Check sheet for the modelled part. Datum: model origin and axes. Units: mm. A direction names the side the tool comes from. Give positions to 0.01 mm unless a question says otherwise; leave off trailing zeros. Loops run counter-clockwise (first coordinate to the right, second up) from the corner with the lowest first, then second, coordinate; pieces in that order, holes last. Notation, with made-up numbers: (-27, 42) -> (-3, 42) arc R9 ccw to (-3, 51) -> close; hole circle Ø4 at (28, -16.75). An arc over 180 degrees is marked (long way). Write each question's results on one line, items separated by ' | '. Start each with the question number.
Item 1: Access from +Z, -Z, +X, -X, +Y, -Y to the whole of each face (thin tool, end or side, straight path). Record for faces 5 (the face through (-0.96, -8.87, -4.34)), 6 (the face through (-8.807, -14.829, 3.935)).
Item 2: Mould release check, pull along X, two halves, no side actions. Record for faces 1 (the face through (-5, -17.018, 5)), 2 (the face through (-1.38, -21.15, -6.2)), 3 (the face through (3, -12.7, -6)), 4 (the face through (2.264, -14.829, 10.412)): pulls with the +X half, pulls with the -X half, needs draft (parallel to the pull), parting line crosses it, or undercut.
Item 3: Gauge pin test, flat ends, axial feed: pin 1 Ø3 at (x, z) = (4.17, 10.33) entering from -Y; pin 2 Ø4.5 at (x, z) = (-3.74, 10.33) entering from +Y; pin 3 Ø6 at (y, z) = (-4, -9.5) entering from -X; pin 4 Ø4 at (x, y) = (-7.5, -10.5) entering from +Z. Record the tip position at first contact, or that the pin passes through.
Item 4: Cross-section at C-C on x = 0. Enter the section's corners in (y, z) (3 decimals).
Item 5: Cross-section at A-A on z = 0. Enter the section's corners in (x, y) (3 decimals).
Item 6: Cross-section at D-D on x = 10. Enter the section's corners in (y, z), then the cut area to 3 significant figures.
Item 7: Scan lines: line 1 along X through (y, z) = (-4.25, 0.5); line 2 along Z through (x, y) = (0, -9.75) (3 decimals); line 3 along Y through (x, z) = (-2, -1). Record each from-to range of solid material in increasing order.
Item 8: Cross-section at B-B on y = -3. Enter the section's corners in (x, z) (3 decimals), then the cut area to 3 significant figures.
from build123d import *

# Parameters (mm, degrees)
F0_R       = 19.685
F1_DEPTH   = 17.018
F2_R       = 14.605
F3_DEPTH   = 12.7
F4_R       = 1.905
F5_DEPTH   = 21.336
F6_R       = 6.35
F7_DEPTH   = 25.4
F7_FACE_R  = 6.35
F8_DEPTH   = 10.16
F9_R       = 4.445
F10_DEPTH  = 25.4
F10_FACE_R = 4.445
F11_DEPTH  = 7.62


with BuildPart() as f1:
    # F0 (on Front) → F1 (new body)
    with BuildSketch(Plane.XZ):
        Circle(F0_R)
    extrude(amount=F1_DEPTH)

    # F2 (on Front) → F3 (cut)
    with BuildSketch(Plane.XZ):
        Circle(F2_R)
    extrude(amount=F3_DEPTH, mode=Mode.SUBTRACT)

    # F4 (on Front) → F5 (cut)
    with BuildSketch(Plane.XZ):
        with Locations((-3.744667, 10.32798)):
            Circle(F4_R)
        with Locations((-10.624286, 3.362366)):
            Circle(F4_R)
        with Locations((-10.624286, -3.517252)):
            Circle(F4_R)
        with Locations((-3.400686, -10.05289)):
            Circle(F4_R)
        with Locations((3.994903, -10.05289)):
            Circle(F4_R)
        with Locations((11.390493, -3.517252)):
            Circle(F4_R)
        with Locations((4.166894, 10.32798)):
            Circle(F4_R)
        with Locations((11.390493, 3.018385)):
            Circle(F4_R)
    extrude(amount=F5_DEPTH, mode=Mode.SUBTRACT)

    # F6 (on Front) → F7 (join)
    with BuildSketch(Plane.XZ):
        Circle(F6_R)
    extrude(amount=F7_DEPTH)

    # F7_face (on face) → F8 (cut)
    with BuildSketch(Plane(origin=(0, 0, 0), x_dir=(1, 0, 0), z_dir=(0, 1, 0))):
        Circle(F7_FACE_R)
    extrude(amount=-F8_DEPTH, mode=Mode.SUBTRACT)

    # F9 (on Front) → F10 (join)
    with BuildSketch(Plane.XZ):
        Circle(F9_R)
    extrude(amount=F10_DEPTH)

    # F10_face (on face) → F11 (cut)
    with BuildSketch(Plane(origin=(0, 0, 0), x_dir=(1, 0, 0), z_dir=(0, 1, 0))):
        Circle(F10_FACE_R)
    extrude(amount=-F11_DEPTH, mode=Mode.SUBTRACT)


solid = f1.part
Answer sheet:
1) face 5: +Y | face 6: +Y, -Y
2) face 1: needs draft | face 2: parting line crosses it | face 3: undercut | face 4: undercut
3) pin 1: passes through | pin 2: stops at y = -12.7 | pin 3: stops at x = -18.58 | pin 4: stops at z = 18.9
4) outline: (-25.4, -6.35) -> (-17.018, -6.35) -> (-17.018, -19.685) -> (0, -19.685) -> (0, -14.605) -> (-12.7, -14.605) -> (-12.7, -6.35) -> (-10.16, -6.35) -> (-10.16, -4.445) -> (-7.62, -4.445) -> (-7.62, 4.445) -> (-10.16, 4.445) -> (-10.16, 6.35) -> (-12.7, 6.35) -> (-12.7, 14.605) -> (0, 14.605) -> (0, 19.685) -> (-17.018, 19.685) -> (-17.018, 6.35) -> (-25.4, 6.35) -> close
5) outline: (-19.685, -17.018) -> (-6.35, -17.018) -> (-6.35, -25.4) -> (6.35, -25.4) -> (6.35, -17.018) -> (19.685, -17.018) -> (19.685, 0) -> (14.605, 0) -> (14.605, -12.7) -> (6.35, -12.7) -> (6.35, -10.16) -> (4.445, -10.16) -> (4.445, -7.62) -> (-4.445, -7.62) -> (-4.445, -10.16) -> (-6.35, -10.16) -> (-6.35, -12.7) -> (-14.605, -12.7) -> (-14.605, 0) -> (-19.685, 0) -> close
6) outline: (-17.02, -16.96) -> (0, -16.96) -> (0, -10.64) -> (-12.7, -10.64) -> (-12.7, -4.82) -> (-17.02, -4.82) -> close; (-17.02, -2.22) -> (-12.7, -2.22) -> (-12.7, 1.72) -> (-17.02, 1.72) -> close; (-17.02, 4.32) -> (-12.7, 4.32) -> (-12.7, 10.64) -> (0, 10.64) -> (0, 16.96) -> (-17.02, 16.96) -> close | area: 284 mm²
7) line 1: x = -19.68 to -14.6, 14.6 to 19.68 | line 2: z = -19.685 to -14.605, -4.445 to 4.445, 14.605 to 19.685 | line 3: y = -25.4 to -7.62
8) outline: circle Ø39.37 at (0, 0); hole circle Ø29.21 at (0, 0) | area: 547 mm²
